CAD build for the part. Positions are in the model's coordinates, mm. Face numbers are marked on the shaded views. A direction names the side the tool comes from. Give positions to 0.01 mm unless a question says otherwise; leave off trailing zeros. Write each loop counter-clockwise with the first axis right and the second up, starting at its lowest first coordinate (ties: lowest second). Pieces come first, ordered by that corner, then holes. Notation, with made-up numbers: (57, 37.25) -> (102, 37.25) arc R24 ccw to (102, 48.25) -> close; hole circle Ø9 at (-13.5, 8.5). An arc over 180 degrees is marked (long way). Answer in a Markdown table with one row per item. Add a question column.
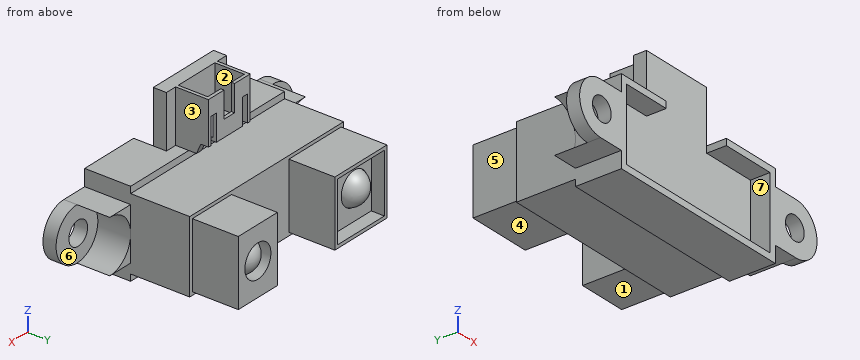
```python
from build123d import *

# Parameters (mm, degrees)
EXTRUDE_1_DEPTH     = 7
CUT_EXTRUDE_START   = -5
SKETCH_2_R          = 4
CUT_EXTRUDE_1_DEPTH = 5
SKETCH_3_W          = 29.5
SKETCH_3_H          = 11
EXTRUDE_2_DEPTH     = 9
SKETCH_4_W          = 7.5
SKETCH_4_H          = 10
SKETCH_4_W_2        = 10
EXTRUDE_3_DEPTH     = 7
SKETCH_5_W          = 9
SKETCH_5_H          = 9
CUT_EXTRUDE_2_DEPTH = 2
SKETCH_6_R          = 2.5
CUT_EXTRUDE_3_DEPTH = 2.2
SKETCH_7_R          = 1.796075295
CUT_EXTRUDE_4_DEPTH = 45.902672526
SKETCH_8_W          = 11.533749137
SKETCH_8_H          = 5
EXTRUDE_4_DEPTH     = 8
CUT_EXTRUDE_5_DEPTH = 3
SKETCH_11_W         = 8
SKETCH_11_H         = 6.5
EXTRUDE_6_DEPTH     = 5
EXTRUDE_7_DEPTH     = 1
EXTRUDE_8_DEPTH     = 1
CUT_EXTRUDE_6_DEPTH = 4
SKETCH_15_W         = 7
SKETCH_15_H         = 4.5
CUT_EXTRUDE_7_DEPTH = 2
SKETCH_16_W         = 1
SKETCH_16_H         = 4
CUT_EXTRUDE_8_DEPTH = 1


# Read off the part's stored shape, not the designer's step: 圆顶1, 圆顶2
with BuildPart() as part:
    # 草图1 → 凸台-拉伸1 (new body)
    with BuildSketch(Plane(origin=(0, 0, 0), x_dir=(1, 0, 0), z_dir=(0, 1, 0))):
        with BuildLine():
            Line((0, 0), (29.5, 0))
            Line((29.5, 0), (29.5, -2.5))
            Line((29.5, -2.5), (33.5, -2.5))
            ThreePointArc((33.5, -2.5), (37.5, -6.5), (33.5, -10.5))
            Line((33.5, -10.5), (29.5, -10.5))
            Line((29.5, -10.5), (29.5, -13))
            Line((29.5, -13), (0, -13))
            Line((0, -13), (0, -10.5))
            Line((0, -10.5), (-4, -10.5))
            ThreePointArc((-4, -10.5), (-8, -6.5), (-4, -2.5))
            Line((-4, -2.5), (0, -2.5))
            Line((0, -2.5), (0, 0))
        make_face()
    extrude(amount=EXTRUDE_1_DEPTH)

    # 草图2 → 切除-拉伸1 (cut)
    with BuildSketch(Plane(origin=(0, 7, 0), x_dir=(1, 0, 0), z_dir=(0, 1, 0)).offset(CUT_EXTRUDE_START)):
        with Locations((-4, -6.5)):
            Circle(SKETCH_2_R)
        with Locations((33.5, -6.5)):
            Circle(SKETCH_2_R)
    extrude(amount=CUT_EXTRUDE_1_DEPTH, mode=Mode.SUBTRACT)

    # 草图3 → 凸台-拉伸2 (add)
    with BuildSketch(Plane(origin=(0, 7, 0), x_dir=(1, 0, 0), z_dir=(0, 1, 0))):
        with Locations((14.75, -6.5)):
            Rectangle(SKETCH_3_W, SKETCH_3_H)
    extrude(amount=EXTRUDE_2_DEPTH)

    # 草图4 → 凸台-拉伸3 (add)
    with BuildSketch(Plane(origin=(0, 16, 0), x_dir=(1, 0, 0), z_dir=(0, 1, 0))):
        with Locations((25.25, -6.5)):
            Rectangle(SKETCH_4_W, SKETCH_4_H)
        with Locations((5.5, -6.5)):
            Rectangle(SKETCH_4_W_2, SKETCH_4_H)
    extrude(amount=EXTRUDE_3_DEPTH)

    # 草图5 → 切除-拉伸2 (cut)
    with BuildSketch(Plane(origin=(0, 23, 0), x_dir=(1, 0, 0), z_dir=(0, 1, 0))):
        with Locations((5.5, -6.5)):
            Rectangle(SKETCH_5_W, SKETCH_5_H)
    extrude(amount=-CUT_EXTRUDE_2_DEPTH, mode=Mode.SUBTRACT)

    # 草图6 → 切除-拉伸3 (cut)
    with BuildSketch(Plane(origin=(0, 23, 0), x_dir=(1, 0, 0), z_dir=(0, 1, 0))):
        with Locations(Location((25.25, -6.5, 0), (0, 0, 270))):
            Circle(SKETCH_6_R)
        with Locations(Location((4.253331237, -6.5, 0), (0, 0, 270))):
            Circle(SKETCH_6_R)
    extrude(amount=-CUT_EXTRUDE_3_DEPTH, mode=Mode.SUBTRACT)

    # 圆顶1 outline → 圆顶1 (revolve)
    with BuildSketch(Plane(origin=(4.253331237, 0, 6.5), x_dir=(1, 0, 0), z_dir=(0, 0, 1))):
        with BuildLine():
            Line((0, 20.8), (2.500000001, 20.799999998))
            ThreePointArc((2.500000001, 20.799999998), (1.60078106, 22.238476323), (0, 22.8))
            Line((0, 22.8), (0, 20.8))
        make_face()
    revolve(axis=Axis((4.253331237, 0, 6.5), (0, 1, 0)))

    # 圆顶2 outline → 圆顶2 (revolve)
    with BuildSketch(Plane(origin=(25.25, 0, 6.5), x_dir=(1, 0, 0), z_dir=(0, 0, 1))):
        with BuildLine():
            Line((0, 20.8), (2.500000001, 20.799999997))
            ThreePointArc((2.500000001, 20.799999997), (1.60078106, 22.238476323), (0, 22.8))
            Line((0, 22.8), (0, 20.8))
        make_face()
    revolve(axis=Axis((25.25, 0, 6.5), (0, 1, 0)))

    # 草图7 → 切除-拉伸4 (cut, through all)
    with BuildSketch(Plane(origin=(0, 2, 0), x_dir=(1, 0, 0), z_dir=(0, 1, 0))):
        with Locations(Location((-3.75, -6.5, 0), (0, 0, 270))):
            Circle(SKETCH_7_R)
        with Locations(Location((33.25, -6.5, 0), (0, 0, 270))):
            Circle(SKETCH_7_R)
    extrude(amount=-CUT_EXTRUDE_4_DEPTH, mode=Mode.SUBTRACT)

    # 草图8 → 凸台-拉伸4 (add)
    with BuildSketch(Plane.XY.offset(13)):
        with Locations((14.355989937, 2.5)):
            Rectangle(SKETCH_8_W, SKETCH_8_H)
    extrude(amount=EXTRUDE_4_DEPTH)

    # 草图10 → 切除-拉伸5 (cut)
    with BuildSketch(Plane.XZ):
        Polygon((8.589115368, 21), (8.589115368, 12), (1, 12), (1, 1), (28.5, 1), (28.5, 12), (20.122864505, 12), (20.122864505, 21), align=None)
    extrude(amount=-CUT_EXTRUDE_5_DEPTH, mode=Mode.SUBTRACT)

    # 草图11 → 凸台-拉伸6 (add)
    with BuildSketch(Plane(origin=(0, 5, 0), x_dir=(1, 0, 0), z_dir=(0, 1, 0))):
        with Locations((14.355989936, -17.75)):
            Rectangle(SKETCH_11_W, SKETCH_11_H)
    extrude(amount=EXTRUDE_6_DEPTH)

    # 草图12 → 凸台-拉伸7 (add)
    with BuildSketch(Plane(origin=(18.355989936, 0, 0), x_dir=(0, 0, -1), z_dir=(1, 0, 0))):
        Polygon((-14.5, 8.832927064), (-13, 8.172497524), (-13, 5), (-14.5, 5), align=None)
    extrude(amount=-EXTRUDE_7_DEPTH)

    # 草图13 → 凸台-拉伸8 (add)
    with BuildSketch(Plane.ZY.offset(-10.355989936)):
        Polygon((14.5, 8.832927064), (13, 8.172497524), (13, 5), (14.5, 5), align=None)
    extrude(amount=-EXTRUDE_8_DEPTH)

    # 草图14 → 切除-拉伸6 (cut)
    with BuildSketch(Plane.XY.offset(21)):
        Polygon((10.855989936, 5), (17.855989936, 5), (17.855989936, 9.5), (15.355989936, 9.5), (15.355989936, 10), (13.355989936, 10), (13.355989936, 9.5), (10.855989936, 9.5), align=None)
    extrude(amount=-CUT_EXTRUDE_6_DEPTH, mode=Mode.SUBTRACT)

    # 草图15 → 切除-拉伸7 (cut)
    with BuildSketch(Plane.XY.offset(17)):
        with Locations((14.355989936, 7.25)):
            Rectangle(SKETCH_15_W, SKETCH_15_H)
    extrude(amount=-CUT_EXTRUDE_7_DEPTH, mode=Mode.SUBTRACT)

    # 草图16 → 切除-拉伸8 (cut)
    with BuildSketch(Plane(origin=(0, 10, 0), x_dir=(1, 0, 0), z_dir=(0, 1, 0))):
        with Locations((11.355989936, -16.5)):
            Rectangle(SKETCH_16_W, SKETCH_16_H)
        with Locations((17.355989936, -16.5)):
            Rectangle(SKETCH_16_W, SKETCH_16_H)
    extrude(amount=-CUT_EXTRUDE_8_DEPTH, mode=Mode.SUBTRACT)


solid = part.part
```
Item 1: Which spindle directions (+Z, -Z, +X, -X, +Y, -Y) get a long thin tool onto all of the face, cutting with end or side? Do the marked faces 4, 5, 6 and 7. Say none if no direction does.
Item 2: Mould opens along X. For the marked faces 1, 2 and 3 say: released by +X, released by -X, zero draft, split by the parting line, or undercut.
Item 3: Slice it at D-D, the plane y = 4.5. List the corners of the cut face in (x, z).
Item 4: Probe L1, parallel to X at y = 1.05, z = 6.5; L2, parallel to Z at x = 25.25, y = 22.05; L3, parallel to X at y = 21.6, z = 6.5. List the from-to ranges inside material, lowest first. Write a range as from..to.
Item 5: Slice it at B-B, the plane y = 17.75. List the corners of the cut face in (x, z).
Item 6: Drop flat-ended pins along their axis: pin 1 Ø8 at (y, z) = (20.5, 14) entering from +X; pin 2 Ø1.5 at (x, z) = (21.5, 14.5) entering from -Y; pin 3 Ø4 at (x, z) = (-3.75, 6.5) entering from -Y; pin 4 Ø1 at (x, y) = (25.5, 18.5) entering from +Z. Give the stop position or say it passes through.
Item 7: Slice it at C-C, the plane x = 25.25. List the corners of the cut face in (y, z) (1 decimal).
Item 8: Slice it at A-A, the plane z = 15.75. List the corners of the cut face in (x, y).
Answer key:
| question | item | result |
|---|---|---|
| 1 | face 4 | -Z, +X, -X, +Y |
| 1 | face 5 | +Z, -Z, -X, +Y |
| 1 | face 6 | +X, +Y |
| 1 | face 7 | -Y |
| 2 | face 1 | zero draft |
| 2 | face 2 | undercut |
| 2 | face 3 | released by +X |
| 3 | outline | (-4, 2.5) -> (0, 2.5) -> (0, 0) -> (29.5, 0) -> (29.5, 2.5) -> (33.5, 2.5) arc R4 cw to (33.5, 10.5) -> (29.5, 10.5) -> (29.5, 13) -> (20.12, 13) -> (20.12, 21) -> (8.59, 21) -> (8.59, 13) -> (0, 13) -> (0, 10.5) -> (-4, 10.5) arc R4 cw to start |
| 4 | L1 | x = -8..-5.55, -1.95..1, 28.5..31.45, 35.05..37.5 |
| 4 | L2 | z = 1.5..4, 4.69..8.31, 9..11.5 |
| 4 | L3 | x = 0.5..1, 2.08..6.42, 10..10.5, 21.5..22.75, 23.08..27.42, 27.75..29 |
| 5 | outline | (0.5, 1.5) -> (10.5, 1.5) -> (10.5, 11.5) -> (0.5, 11.5) -> close; (21.5, 1.5) -> (29, 1.5) -> (29, 11.5) -> (21.5, 11.5) -> close |
| 6 | pin 1 | stops at x = 29 |
| 6 | pin 2 | passes through |
| 6 | pin 3 | stops at y = 0 |
| 6 | pin 4 | stops at z = 11.5 |
| 7 | outline | (0, 0) -> (7, 0) -> (7, 1) -> (16, 1) -> (16, 1.5) -> (23, 1.5) -> (23, 4) -> (20.8, 4) arc R2.6 ccw to (20.8, 9) -> (23, 9) -> (23, 11.5) -> (16, 11.5) -> (16, 12) -> (7, 12) -> (7, 13) -> (0, 13) -> (0, 12) -> (3, 12) -> (3, 1) -> (0, 1) -> close |
| 8 | outline | (8.59, 3) -> (20.12, 3) -> (20.12, 5) -> (18.36, 5) -> (18.36, 10) -> (17.86, 10) -> (17.86, 5) -> (10.86, 5) -> (10.86, 10) -> (10.36, 10) -> (10.36, 5) -> (8.59, 5) -> close; (11.86, 9.5) -> (16.86, 9.5) -> (16.86, 10) -> (11.86, 10) -> close |
